from build123d import *

# Parameters (mm, degrees)
BASE_DEPTH = 555.3837


with BuildPart() as part:
    # Sketch1 → Base (new body, symmetric)
    with BuildSketch(Plane.XY):
        with BuildLine():
            Line((-377.5837, 12.7), (-377.5837, 288.6837))
            ThreePointArc((-377.5837, 288.6837), (-382.304054982, 300.079645018), (-393.7, 304.8))
            Line((-393.7, 304.8), (-419.1, 304.8))
            Line((-419.1, 304.8), (-419.1, 301.3837))
            Line((-419.1, 301.3837), (-393.7, 301.3837))
            ThreePointArc((-393.7, 301.3837), (-384.719743879, 297.663956121), (-381, 288.6837))
            Line((-381, 288.6837), (-381, 12.7))
            ThreePointArc((-381, 12.7), (-377.280256121, 3.719743879), (-368.3, 0))
            Line((-368.3, 0), (368.3, 0))
            ThreePointArc((368.3, 0), (377.280256121, 3.719743879), (381, 12.7))
            Line((381, 12.7), (381, 288.6837))
            ThreePointArc((381, 288.6837), (384.719743879, 297.663956121), (393.7, 301.3837))
            Line((393.7, 301.3837), (419.1, 301.3837))
            Line((419.1, 301.3837), (419.1, 304.8))
            Line((419.1, 304.8), (393.7, 304.8))
            ThreePointArc((393.7, 304.8), (382.304054982, 300.079645018), (377.5837, 288.6837))
            Line((377.5837, 288.6837), (377.5837, 12.7))
            ThreePointArc((377.5837, 12.7), (374.864567225, 6.135432775), (368.3, 3.4163))
            Line((368.3, 3.4163), (-368.3, 3.4163))
            ThreePointArc((-368.3, 3.4163), (-374.864567225, 6.135432775), (-377.5837, 12.7))
        make_face()
    extrude(amount=BASE_DEPTH, both=True)


solid = part.part
Check sheet for the modelled part. Datum: model origin and axes. Units: mm. A direction names the side the tool comes from. Coordinates: 2 decimals unless noted, no trailing zeros. Loops run counter-clockwise (first coordinate to the right, second up) from the corner with the lowest first, then second, coordinate; pieces in that order, holes last. Notation, with made-up numbers: (48, -5.75) -> (58, -5.75) arc R12 cw to (58, 10.25) -> close; hole circle Ø2 at (-10.75, 67.25). An arc over 180 degrees is marked (long way). Answer in a Markdown table with one row per item.
1. Material ranges on line 1 along X through (y, z) = (206, 392); line 2 along Y through (x, z) = (-110, -371), recorded low to high. Write a range as [from, to].
Check values:
| item | result |
|---|---|
| line 1 | x = [-381, -377.58], [377.58, 381] |
| line 2 | y = [0, 3.42] |
2. Sectioned sample at C-C, the plane x = 238. Record the boundary of the cut face in (y, z).
Check values:
| item | result |
|---|---|
| outline | (0, -555.38) -> (3.42, -555.38) -> (3.42, 555.38) -> (0, 555.38) -> close |
3. Access from +Z, -Z, +X, -X, +Y, -Y to the whole of each face (thin tool, end or side, straight path). Record for faces 1 (the face through (406, 301.384, 8)), 2 (the face through (377.584, 153, 8)), 3 (the face through (-407, 301.384, 8)).
Check values:
| item | result |
|---|---|
| face 1 | +Z, -Z, +X, -Y |
| face 2 | +Z, -Z, +Y |
| face 3 | +Z, -Z, -X, -Y |
4. Sectioned sample at A-A, the plane y = 239. Record the boundary of the cut face in (x, z).
Check values:
| item | result |
|---|---|
| outline | (-381, -555.38) -> (-377.58, -555.38) -> (-377.58, 555.38) -> (-381, 555.38) -> close; (377.58, -555.38) -> (381, -555.38) -> (381, 555.38) -> (377.58, 555.38) -> close |
5. Sectioned sample at B-B, the plane z = 422. Record the boundary of the cut face in (x, y), then the cut area to 3 significant figures.
Check values:
| item | result |
|---|---|
| outline | (-419.1, 301.38) -> (-393.7, 301.38) arc R12.7 cw to (-381, 288.68) -> (-381, 12.7) arc R12.7 ccw to (-368.3, 0) -> (368.3, 0) arc R12.7 ccw to (381, 12.7) -> (381, 288.68) arc R12.7 cw to (393.7, 301.38) -> (419.1, 301.38) -> (419.1, 304.8) -> (393.7, 304.8) arc R16.12 ccw to (377.58, 288.68) -> (377.58, 12.7) arc R9.28 cw to (368.3, 3.42) -> (-368.3, 3.42) arc R9.28 cw to (-377.58, 12.7) -> (-377.58, 288.68) arc R16.12 ccw to (-393.7, 304.8) -> (-419.1, 304.8) -> close |
| area | 4,850 mm2 |
6. Go/stop test with flat-tipped pins: pin 1 (8 mm diameter, centred on x = 311.5, z = 119.5, fed in from +Y); pin 2 (12.5 mm diameter, centred on x = 407.5, z = -238, fed in from -Y); pin 3 (2 mm diameter, centred on y = 97, z = -295, fed in from +X). Record where each tip stops, or that it passes through.
Check values:
| item | result |
|---|---|
| pin 1 | stops at y = 3.42 |
| pin 2 | stops at y = 301.38 |
| pin 3 | stops at x = 381 |
